```python
from build123d import *

# Parameters (mm, degrees)
F0_W           = 101.6
F0_H           = 101.6
F1_DEPTH       = 25.4
F2_W           = 76.2
F2_H           = 76.2
F7_D           = 12.7
F7_DEPTH       = 25.4
F7_TIP         = 3.8154649308
F9_D           = 19.05
F9_DEPTH       = 76.2
F9_CBORE_D     = 20.32
F9_CBORE_DEPTH = 10.16
F9_TIP         = 5.7231973962


with BuildPart() as f1:
    # F0 (on Front) → F1 (new body)
    with BuildSketch(Plane.XZ):
        with Locations((50.8, 50.8)):
            Rectangle(F0_W, F0_H)
    extrude(amount=F1_DEPTH)

    # F4 (on offset) → F5 section 0
    with BuildSketch(Plane.XZ.offset(349.25)):
        Polygon((50.8, 88.9), (12.7, 50.8), (50.8, 12.7), (88.9, 50.8), align=None)
    # F2 (on face) → F5 section 1
    with BuildSketch(Plane.XZ.offset(25.4)):
        with Locations((50.8, 50.8)):
            Rectangle(F2_W, F2_H)
    loft()

    # F7
    with Locations(Plane(origin=(0, 0, 0), x_dir=(-1, 0, 0), z_dir=(0, 1, 0))):
        with Locations((-50.8, 50.8)):
            Hole(F7_D / 2, depth=F7_DEPTH)
            with Locations((0, 0, -(F7_DEPTH + F7_TIP / 2))):  # 118° drill point
                Cone(0, F7_D / 2, F7_TIP, mode=Mode.SUBTRACT)

    # F9
    with Locations(Plane.XZ.offset(349.25)):
        with Locations((50.6945904344, 50.7964529097)):
            CounterBoreHole(F9_D / 2, F9_CBORE_D / 2, F9_CBORE_DEPTH, depth=F9_DEPTH)
            with Locations((0, 0, -(F9_DEPTH + F9_TIP / 2))):  # 118° drill point
                Cone(0, F9_D / 2, F9_TIP, mode=Mode.SUBTRACT)


solid = f1.part
```
Geometry: final body of the model. Coordinates: model frame, mm. A direction names the side the tool comes from. Coordinates: 2 decimals unless noted, no trailing zeros. Order: outer loops, then holes, each group sorted by start corner. A loop starts at its lowest first (then second) coordinate and runs counter-clockwise, first axis right, second up. Notation, with made-up numbers: (51.5, 25) - (81.5, 25) arc R4 ccw to (81.5, 29) - close; hole circle Ø9 at (75, 60). An arc over 180 degrees is marked (long way). Write each question's results on one line, items separated by ' | '.
1) Section A-A, the plane x = 7.5. Return loops of the section in (y, z), plus the area to 3 significant figures.
Results list:
outline: (-25.4, 0) - (0, 0) - (0, 101.6) - (-25.4, 101.6) - close | area: 2,580 mm^2
2) Set-up query: faces 1 (the flat face through (60, -349.25, 43)), 2 (the cylindrical face through (56.857, -12.878, 52.707)), 3 (the cylindrical face through (52.76, -305.61, 41.5)). Return all of +Z, -Z, +X, -X, +Y, -Y with unobstructed straight access to the full face (end or side cutting, diameter ignored); none if empty.
Results list:
face 1: +Z, -Z, +X, -X, -Y | face 2: +Y | face 3: -Y
3) Pin query (flat end, axial travel): pin 1 (1 mm diameter, centred on y = -290, z = 13.5, fed in from +X); pin 2 (10 mm diameter, centred on x = 49, z = 46, fed in from -Y); pin 3 (3 mm diameter, centred on y = -279, z = 71.5, fed in from +X). Return the tip coordinate at first contact, or that it passes through.
Results list:
pin 1: x = 58.67 | pin 2: y = -339.09 | pin 3: x = 71.91
4) Pull-direction query (Z, two-part tool) for faces 4 (the flat face through (50, -13, 0)), 5 (the flat face through (61, 0, 52)), 6 (the conical face through (50.944, -28.553, 51.893)), 7 (the flat face through (50, -13, 101.6)); classes: pulls with the +Z half, pulls with the -Z half, needs draft (parallel to the pull), parting line crosses it, or undercut.
Results list:
face 4: pulls with the -Z half | face 5: needs draft | face 6: undercut | face 7: pulls with the +Z half
5) Line query: line 1 (Y direction, x = 95, z = 14); line 2 (X direction, y = -39, z = 83.5); line 3 (Z direction, x = 77.5, y = -318). Output: solid intervals per line, ascending. Write a range as from..to.
Results list:
line 1: -25.4..0 | line 2: 14.18..88.82 | line 3: 40.64..63.87
